Autodesk Inventor part; units mm, degrees
ref_plane "YZ Plane" through (0, 0, 0) normal (1, 0, 0) x (0, 1, 0)
ref_plane "XZ Plane" through (0, 0, 0) normal (0, 1, 0) x (-1, 0, 0)
ref_plane "XY Plane" through (0, 0, 0) normal (0, 0, 1) x (1, 0, 0)
sketch "Sketch1" plane through (0, 0, 0) normal (0, 0, 1) x (1, 0, 0)
  line L0 (0, 0) -> (-80, 0)
  line L1 (-80, 0) -> (-80, 358)
  line L2 (-80, 358) -> (0, 358)
  line L3 (0, 358) -> (0, 0)
  dimension "d0" = 80
  dimension "d1" = 358
extrude "Extrusion1" add sketch "Sketch1" along normal blind 15
sketch "Sketch2" plane through (0, 0, 15) normal (0, 0, 1) x (1, 0, 0)
  line L0 (-80, 0) -> (0, 0)
  line L1 (-80, 0) -> (-55, 0)
  line L2 (-55, 0) -> (-55, 50)
  line L3 (-55, 50) -> (-80, 50)
  line L4 (-80, 50) -> (-80, 0)
  dimension "d4" = 25
  dimension "d5" = 50
extrude "Extrusion2" cut sketch "Sketch2" against normal through all
ref_plane "Work Plane1" through (0, 179, 0) normal (0, -1, 0) x (1, 0, 0)
mirror "Mirror1" about plane through (0, 179, 0) normal (0, -1, 0) of "Extrusion2"
properties part number "MPX-rib" material "Wood (Cherry)"
Verification items for the finished model (mm, model axes). A direction names the side the tool comes from. Give positions to 0.01 mm unless a question says otherwise; leave off trailing zeros. Loops run counter-clockwise (first coordinate to the right, second up) from the corner with the lowest first, then second, coordinate; pieces in that order, holes last.
1. Material ranges on probe 1 along Y at (x, z) = (-65.5, 10.25); probe 2 along X at (y, z) = (35.5, 7.25), recorded low to high.
Derived:
probe 1: y = 50 to 308
probe 2: x = -55 to 0
2. Cross-section at C-C on x = -66. Record the cut outline in (y, z), and give its area (3 significant figures).
Derived:
outline: (50, 0) - (308, 0) - (308, 15) - (50, 15) - close
area: 3,870 mm2
3. Cross-section at B-B on y = 44.5. Record the cut outline in (x, z).
Derived:
outline: (-55, 0) - (0, 0) - (0, 15) - (-55, 15) - close
4. Cross-section at A-A on z = 6. Record the cut outline in (x, y), and give its area (3 significant figures).
Derived:
outline: (-80, 50) - (-55, 50) - (-55, 0) - (0, 0) - (0, 358) - (-55, 358) - (-55, 308) - (-80, 308) - close
area: 26,100 mm2
5. Go/stop test with flat-tipped pins: P1, Ø7.5, axis at x = -71, z = 8, coming from the +Y side; P2, Ø4.5, axis at x = -65.5, z = 9.5, coming from the -Y side; P3, Ø4.5, axis at y = 323, z = 9.5, coming from the -X side. Record where each tip stops, or that it passes through.
Derived:
P1: stops at y = 308
P2: stops at y = 50
P3: stops at x = -55
6. Tool access check on faces 1 (the flat face through (-27, 0, 7)), 2 (the flat face through (-55, 25, 8)), 3 (the flat face through (-68, 308, 8)). Record the directions out of +Z, -Z, +X, -X, +Y, -Y that give a thin tool (end or side, any length) a straight path to the whole face; none if there is none.
Derived:
face 1: +Z, -Z, +X, -X, -Y
face 2: +Z, -Z, -X, -Y
face 3: +Z, -Z, -X, +Y
